Part model, mm, in its own coordinate system. Face numbers are marked on the shaded views. A direction names the side the tool comes from. Coordinates: 2 decimals unless noted, no trailing zeros. Write each loop counter-clockwise with the first axis right and the second up, starting at its lowest first coordinate (ties: lowest second). Pieces come first, ordered by that corner, then holes. Notation, with made-up numbers: (33.5, -14.75) -> (41.5, -14.75) arc R19 cw to (41.5, 6.25) -> close; hole circle Ø6 at (-17, -17.75). An arc over 180 degrees is marked (long way). One line per question, with ' | ' between items. Start each with the question number.
Item 1: Two-plate mould, pull along X, no slides. Class the marked faces 1, 2, 3 and 4: pulls with the +X half, pulls with the -X half, needs draft (parallel to the pull), parting line crosses it, or undercut.
Item 2: Saw through at D-D (y = 22.5). List the corners of the cut face in (x, z).
Item 3: Saw through at C-C (x = 12). List the corners of the cut face in (y, z), and give its area (3 significant figures).
Item 4: 3-axis set-ups, long thin cutter, end or side, ignore diameter. For the marked faces 5, 6 and 7: which of +Z, -Z, +X, -X, +Y, -Y reach the whole face in a straight line?
Item 5: Saw through at B-B (z = -3). Count the separate pieces of the cut face and the enclosed holes in it, and give its area (3 significant figures).
Item 6: Pin check, flat tip, straight feed: pin 1 (5 mm diameter, centred on x = 9.52, y = 46.04, fed in from +Z). Stop position of the tip, or through.
Item 7: Saw through at A-A (y = 16). List the corners of the cut face in (x, z).
Item 8: Probe probe 1 along Y at (x, z) = (10.5, -4); probe 2 along Y at (x, z) = (10.75, -4.5); probe 3 along X at (y, z) = (17, -1.5). List the from-to ranges inside material, lowest first. Write a range as [from, to].
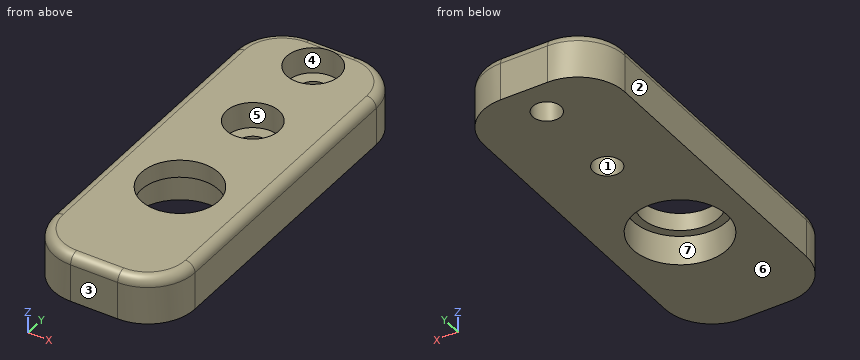
from build123d import *

# Parameters (mm, degrees)
SKETCH1_W                                      = 6.35
SKETCH1_H                                      = 50.8
BODY_DEPTH                                     = 19.05
SKETCH2_R                                      = 5.207
PITCH_AXLE_OPENING_DEPTH                       = 6.35
CBORE_FOR_6_SOCKET_HEAD_CAP_SCREW1_D           = 3.7973
CBORE_FOR_6_SOCKET_HEAD_CAP_SCREW1_CBORE_D     = 7.14502
CBORE_FOR_6_SOCKET_HEAD_CAP_SCREW1_CBORE_DEPTH = 3.5052
FILLET1_R                                      = 6.35
FILLET2_R                                      = 1.27
SKETCH2_3_R                                    = 6.35
SKETCH2_3_R_2                                  = 5.207
BEARING_RECESS_DEPTH                           = 3.96748


with BuildPart() as part:
    # Sketch1 → Body (new body)
    with BuildSketch(Plane(origin=(0, 0, 0), x_dir=(0, 0, -1), z_dir=(1, 0, 0))):
        with Locations((3.175, 25.4)):
            Rectangle(SKETCH1_W, SKETCH1_H)
    extrude(amount=BODY_DEPTH)

    # Sketch2 → Pitch Axle Opening (cut)
    with BuildSketch(Plane(origin=(0, 0, -6.35), x_dir=(-1, 0, 0), z_dir=(0, 0, -1))):
        with Locations((-9.525, 18.034)):
            Circle(SKETCH2_R)
    extrude(amount=-PITCH_AXLE_OPENING_DEPTH, mode=Mode.SUBTRACT)

    # CBORE for #6 Socket Head Cap Screw1 (through all)
    with Locations(Plane.XY):
        with Locations((9.525, 46.0375), (9.525, 33.3375)):
            CounterBoreHole(CBORE_FOR_6_SOCKET_HEAD_CAP_SCREW1_D / 2, CBORE_FOR_6_SOCKET_HEAD_CAP_SCREW1_CBORE_D / 2, CBORE_FOR_6_SOCKET_HEAD_CAP_SCREW1_CBORE_DEPTH)

    # Fillet1
    fillet1_edges = [part.edges().sort_by_distance(p)[0] for p in [
        (19.05, 50.8, -3.175),
        (19.05, 0, -3.175),
        (0, 50.8, -3.175),
        (0, 0, -3.175),
    ]]
    fillet(fillet1_edges, radius=FILLET1_R)

    # Fillet2
    # the kernel refuses this fillet: 1.27 mm, written as the material it takes off along each edge
    with BuildSketch(Plane(origin=(6.35, 50.8, 0), x_dir=(0, -1, 0), z_dir=(1, 0, 0))) as fillet2_piece_1:
        with BuildLine():
            CenterArc((FILLET2_R, FILLET2_R), FILLET2_R, 180, 90)
            Line((0, FILLET2_R), (0, 0))
            Line((0, 0), (FILLET2_R, 0))
        make_face()
    extrude(amount=6.35, mode=Mode.SUBTRACT)
    with BuildSketch(Plane(origin=(0, 6.35, 0), x_dir=(1, 0, 0), z_dir=(0, 1, 0))) as fillet2_piece_2:
        with BuildLine():
            CenterArc((FILLET2_R, FILLET2_R), FILLET2_R, 180, 90)
            Line((0, FILLET2_R), (0, 0))
            Line((0, 0), (FILLET2_R, 0))
        make_face()
    extrude(amount=38.1, mode=Mode.SUBTRACT)
    with BuildSketch(Plane(origin=(6.35, 0, 0), x_dir=(0, 1, 0), z_dir=(1, 0, 0))) as fillet2_piece_3:
        with BuildLine():
            CenterArc((FILLET2_R, -FILLET2_R), FILLET2_R, 90, 90)
            Line((0, -FILLET2_R), (0, 0))
            Line((0, 0), (FILLET2_R, 0))
        make_face()
    extrude(amount=6.35, mode=Mode.SUBTRACT)
    with BuildSketch(Plane(origin=(19.05, 6.35, 0), x_dir=(-1, 0, 0), z_dir=(0, 1, 0))) as fillet2_piece_4:
        with BuildLine():
            CenterArc((FILLET2_R, -FILLET2_R), FILLET2_R, 90, 90)
            Line((0, -FILLET2_R), (0, 0))
            Line((0, 0), (FILLET2_R, 0))
        make_face()
    extrude(amount=38.1, mode=Mode.SUBTRACT)
    with BuildSketch(Plane(origin=(12.7, 6.35, 0), x_dir=(0, -1, 0), z_dir=(-1, 0, 0))) as fillet2_piece_5:
        with BuildLine():
            CenterArc((6.35 - FILLET2_R, -FILLET2_R), FILLET2_R, 0, 90)
            Line((6.35, -FILLET2_R), (6.35, 0))
            Line((6.35, 0), (6.35 - FILLET2_R, 0))
        make_face()
    revolve(axis=Axis((12.7, 6.35, 0), (0, 0, 1)), revolution_arc=90, mode=Mode.SUBTRACT)
    with BuildSketch(Plane(origin=(6.35, 6.35, 0), x_dir=(0, -1, 0), z_dir=(1, 0, 0))) as fillet2_piece_6:
        with BuildLine():
            CenterArc((6.35 - FILLET2_R, FILLET2_R), FILLET2_R, 270, 90)
            Line((6.35, FILLET2_R), (6.35, 0))
            Line((6.35, 0), (6.35 - FILLET2_R, 0))
        make_face()
    revolve(axis=Axis((6.35, 6.35, 0), (0, 0, -1)), revolution_arc=90, mode=Mode.SUBTRACT)
    with BuildSketch(Plane(origin=(12.7, 44.45, 0), x_dir=(1, 0, 0), z_dir=(0, -1, 0))) as fillet2_piece_7:
        with BuildLine():
            CenterArc((6.35 - FILLET2_R, -FILLET2_R), FILLET2_R, 0, 90)
            Line((6.35, -FILLET2_R), (6.35, 0))
            Line((6.35, 0), (6.35 - FILLET2_R, 0))
        make_face()
    revolve(axis=Axis((12.7, 44.45, 0), (0, 0, 1)), revolution_arc=90, mode=Mode.SUBTRACT)
    with BuildSketch(Plane(origin=(6.35, 44.45, 0), x_dir=(-1, 0, 0), z_dir=(0, -1, 0))) as fillet2_piece_8:
        with BuildLine():
            CenterArc((6.35 - FILLET2_R, FILLET2_R), FILLET2_R, 270, 90)
            Line((6.35, FILLET2_R), (6.35, 0))
            Line((6.35, 0), (6.35 - FILLET2_R, 0))
        make_face()
    revolve(axis=Axis((6.35, 44.45, 0), (0, 0, -1)), revolution_arc=90, mode=Mode.SUBTRACT)

    # Sketch2<3> → Bearing Recess (cut)
    with BuildSketch(Plane(origin=(0, 0, -6.35), x_dir=(-1, 0, 0), z_dir=(0, 0, -1))):
        with Locations((-9.525, 18.034)):
            Circle(SKETCH2_3_R)
        with Locations((-9.525, 18.034)):
            Circle(SKETCH2_3_R_2, mode=Mode.SUBTRACT)
    extrude(amount=-BEARING_RECESS_DEPTH, mode=Mode.SUBTRACT)


solid = part.part
From the geometry:
1) face 1: undercut | face 2: pulls with the -X half | face 3: needs draft | face 4: undercut
2) outline: (0, -6.35) -> (5.01, -6.35) -> (5.01, -2.38) -> (6.85, -2.38) -> (6.85, 0) -> (1.27, 0) arc R1.27 ccw to (0, -1.27) -> close; (12.2, -2.38) -> (14.04, -2.38) -> (14.04, -6.35) -> (19.05, -6.35) -> (19.05, -1.27) arc R1.27 ccw to (17.78, 0) -> (12.2, 0) -> close
3) outline: (0, -6.35) -> (12.19, -6.35) -> (12.19, -2.38) -> (13.45, -2.38) -> (13.45, 0) -> (1.27, 0) arc R1.27 ccw to (0, -1.27) -> close; (22.62, -2.38) -> (23.88, -2.38) -> (23.88, -6.35) -> (50.8, -6.35) -> (50.8, -1.27) arc R1.27 ccw to (49.53, 0) -> (48.61, 0) -> (48.61, -3.51) -> (43.46, -3.51) -> (43.46, 0) -> (35.91, 0) -> (35.91, -3.51) -> (30.76, -3.51) -> (30.76, 0) -> (22.62, 0) -> close | area: 218 mm2
4) face 5: +Z | face 6: -Z, +X, -X, +Y, -Y | face 7: -Z
5) separate pieces: 1 | enclosed holes: 3 | area: 726 mm2
6) pin 1: z = -3.51
7) outline: (0, -6.35) -> (3.51, -6.35) -> (3.51, -2.38) -> (4.73, -2.38) -> (4.73, 0) -> (1.27, 0) arc R1.27 ccw to (0, -1.27) -> close; (14.32, -2.38) -> (15.54, -2.38) -> (15.54, -6.35) -> (19.05, -6.35) -> (19.05, -1.27) arc R1.27 ccw to (17.78, 0) -> (14.32, 0) -> close
8) probe 1: [0, 11.76], [24.31, 31.71], [34.97, 44.41], [47.67, 50.8] | probe 2: [0, 11.8], [24.26, 31.89], [34.79, 44.59], [47.49, 50.8] | probe 3: [0, 4.42], [14.63, 19.05]
